The model under review builds one solid part; all positions refer to its coordinate system, in mm. A direction names the side the tool comes from. Round coordinates to 2 decimals unless told otherwise and drop trailing zeros. Order: outer loops, then holes, each group sorted by start corner. A loop starts at its lowest first (then second) coordinate and runs counter-clockwise, first axis right, second up. Notation, with made-up numbers: M 66.25,-0.75 L 110.25,-0.75 A34 ccw 110.25,36.25 Z; hole C 50.25,53.5 d3. An arc over 180 degrees is marked long. Answer as a JSON object with one key per item and string values. Group by question number.
1) Consider section A-A, the plane z = 0. Write out the cut boundary in (x, y), then the cut area to 3 significant figures.
2) Consider section B-B, the plane y = 2. Count the separate pieces of the cut face and the enclosed holes in it, then the cut area to 3 significant figures.
3) Insertion check: pin 1 Ø2 at (x, z) = (1.5, 25.5) entering from -Y; pin 2 Ø0.9 at (y, z) = (2, 28) entering from -X; pin 3 Ø5 at (y, z) = (4.5, 22.5) entering from +X; pin 4 Ø5 at (x, z) = (0.5, 18) entering from +Y. Each pin has a flat end and moves straight along its axis. Give the tip position at first contact, or say it passes through.
4) Consider section D-D, the plane x = -3.5. Write out the cut boundary in (y, z).
5) Consider section C-C, the plane z = 28. Write out the cut boundary in (x, y).
6) To check wall thickness, follow line 1 (X direction, y = 1.05, z = 0); line 2 (Z direction, x = 1.4, y = 2); line 3 (Z direction, x = 0.6, y = 2). State the ranges of each line that lie inside material, in increasing order.
7) For faces 1 (the flat face through (-1.75, 4, 11)), 2 (the flat face through (0, 7, 2)), 3 (the cylindrical face through (1.01, 4.05, 26.53)), list the 3-axis set-ups (+Z, -Z, +X, -X, +Y, -Y) from which the entire face can be reached by the end or side of a thin tool; tool diameter is ignored.
8) The part is to be moulded in two halves that separate along X. For faces 4 (the flat face through (1.75, 3, 17)), 5 (the cylindrical face through (0.173, 1.479, -4.497)), 6 (the cylindrical face through (-0.97, 8.48, -1.27)), 7 (the cylindrical face through (-0.97, 1.48, -1.27)), say which applies: +X half, -X half, draft (parallel to the pull), parting line (faces both ways), or undercut.
```python
from build123d import *

# Parameters (mm, degrees)
SKETCH4_R           = 4.5
SKETCH4_R_2         = 1.6
BOSS_EXTRUDE3_DEPTH = 3
BOSS_EXTRUDE4_START = 4
SKETCH5_R           = 4.5
SKETCH5_R_2         = 1.6
BOSS_EXTRUDE4_DEPTH = 3
BOSS_EXTRUDE5_START = -10
BOSS_EXTRUDE5_DEPTH = 10
CUT_EXTRUDE1_DEPTH  = 17.126453423
SKETCH8_W           = 3.5
SKETCH8_H           = 4
BOSS_EXTRUDE6_DEPTH = 17
SKETCH9_R           = 0.75
CUT_EXTRUDE2_DEPTH  = 31.381943651
SKETCH10_R          = 2.25
SKETCH10_R_2        = 0.75
BOSS_EXTRUDE7_DEPTH = 1.5
FILLET1_R           = 10
FILLET2_R           = 10
FILLET3_R           = 1
SKETCH11_W          = 2
SKETCH11_H          = 2.46221445
CUT_EXTRUDE3_DEPTH  = 33.176272314
CHAMFER2_SIZE       = 4
CHAMFER2_SIZE2      = 1.616104903
CHAMFER3_SIZE       = 0.38
CHAMFER3_SIZE_2     = 1.044041419


with BuildPart() as part:
    # Sketch4 → Boss-Extrude3 (new body)
    with BuildSketch(Plane(origin=(0, 0, 0), x_dir=(1, 0, 0), z_dir=(0, 1, 0))):
        with Locations(Location((0, 0, 0), (0, 0, 270))):
            Circle(SKETCH4_R)
        with Locations(Location((0, 0, 0), (0, 0, 270))):
            Circle(SKETCH4_R_2, mode=Mode.SUBTRACT)
    extrude(amount=BOSS_EXTRUDE3_DEPTH)



with BuildPart() as body_2:
    # Sketch5 → Boss-Extrude4 (new body)
    with BuildSketch(Plane(origin=(0, 3, 0), x_dir=(1, 0, 0), z_dir=(0, 1, 0)).offset(BOSS_EXTRUDE4_START)):
        with Locations(Location((0, 0, 0), (0, 0, 270))):
            Circle(SKETCH5_R)
        with Locations(Location((0, 0, 0), (0, 0, 270))):
            Circle(SKETCH5_R_2, mode=Mode.SUBTRACT)
    extrude(amount=BOSS_EXTRUDE4_DEPTH)


with BuildPart() as part_1:
    add(part.part)

    add(body_2.part)  # Boss-Extrude5 merges body 2
    # Sketch6 → Boss-Extrude5 (add)
    with BuildSketch(Plane(origin=(0, 10, 0), x_dir=(1, 0, 0), z_dir=(0, 1, 0)).offset(BOSS_EXTRUDE5_START)):
        with BuildLine():
            ThreePointArc((1.75, -4.145780988), (0, -4.5), (-1.75, -4.145780988))
            Line((-1.75, -4.145780988), (-1.75, -11))
            Line((-1.75, -11), (1.75, -11))
            Line((1.75, -11), (1.75, -4.145780988))
        make_face()
    extrude(amount=BOSS_EXTRUDE5_DEPTH)

    # Sketch7 → Cut-Extrude1 (cut, through all)
    with BuildSketch(Plane.ZY.offset(1.75)):
        Polygon((4.145780988, 7), (4.145780988, 3), (7.145780988, 3), (9.145780988, 5), (7.145780988, 7), align=None)
    extrude(amount=-CUT_EXTRUDE1_DEPTH, mode=Mode.SUBTRACT)

    # Sketch8 → Boss-Extrude6 (add)
    with BuildSketch(Plane.XY.offset(11)):
        with Locations((0, 2)):
            Rectangle(SKETCH8_W, SKETCH8_H)
    extrude(amount=BOSS_EXTRUDE6_DEPTH)

    # Sketch9 → Cut-Extrude2 (cut, through all)
    with BuildSketch(Plane(origin=(1.75, 0, 0), x_dir=(0, 0, -1), z_dir=(1, 0, 0))):
        with Locations((-28, 2)):
            Circle(SKETCH9_R)
    extrude(amount=-CUT_EXTRUDE2_DEPTH, mode=Mode.SUBTRACT)

    # Sketch10 → Boss-Extrude7 (add)
    with BuildSketch(Plane(origin=(1.75, 0, 0), x_dir=(0, 0, -1), z_dir=(1, 0, 0))):
        with Locations((-28, 2)):
            Circle(SKETCH10_R)
        with Locations((-28, 2)):
            Circle(SKETCH10_R_2, mode=Mode.SUBTRACT)
    extrude(amount=-BOSS_EXTRUDE7_DEPTH)

    # Fillet1
    # the kernel refuses this fillet: 10 mm, written as the material it adds along each edge
    with BuildSketch(Plane(origin=(1.75, 4, 11), x_dir=(0, 1, 0), z_dir=(-1, 0, 0))) as fillet1_piece_1:
        with BuildLine():
            CenterArc((10, -9.16515139), FILLET1_R, 113.578178478, 66.421821522)
            Line((0, -9.16515139), (0, 0))
            Line((0, 0), (6, 0))
        make_face()
    extrude(amount=3.5)
    with BuildSketch(Plane(origin=(0.25, 4, 26.969223594), x_dir=(0, 0, -1), z_dir=(1, 0, 0))) as fillet1_piece_2:
        with BuildLine():
            CenterArc((1.431438044, 10), FILLET1_R, 258.404727341, 11.595272659)
            ThreePointArc((-0.578532936, 0.204081633), (-0.282278366, 0.121850768), (0, 0))
            Line((0, 0), (1.431438044, 0))
        make_face()
    extrude(amount=1.5)
    with BuildSketch(Plane(origin=(0.25, 0, 26.969223594), x_dir=(0, -0.33266579589081224, 0.9430447859165186), z_dir=(1, 0, 0))) as fillet1_piece_3:
        with BuildLine():
            CenterArc((1.976747775, 9.906638335), FILLET1_R, 250.569341445, 11.595272659)
            Line((-1.349910184, 0.476190476), (0, 0))
            ThreePointArc((0, 0), (0.306736724, 0.021006375), (0.613473447, 0))
        make_face()
    extrude(amount=1.5)

    # Fillet2
    fillet2_edges = [part_1.edges().sort_by_distance(p)[0] for p in [
        (0, 10, 11),
    ]]
    fillet(fillet2_edges, radius=FILLET2_R)

    # Fillet3
    fillet3_edges = [part_1.edges().sort_by_distance(p)[0] for p in [
        (0, 7, 7.145780988),
        (0, 5, 9.145780988),
        (0, 3, 7.145780988),
    ]]
    fillet(fillet3_edges, radius=FILLET3_R)

    # Sketch11 → Cut-Extrude3 (cut, through all)
    with BuildSketch(Plane.XZ):
        with Locations((-0.75, 26.768892775)):
            Rectangle(SKETCH11_W, SKETCH11_H)
    extrude(amount=-CUT_EXTRUDE3_DEPTH, mode=Mode.SUBTRACT)

    # Chamfer2
    chamfer2_edges = [part_1.edges().sort_by_distance(p)[0] for p in [
        (-1.75, 2, 25.53778555),
    ]]
    chamfer2_side = [part_1.faces().sort_by_distance(p)[0] for p in [
        (-1.75, 3.550024841, 13.432455859),
    ]]
    chamfer(chamfer2_edges, length=CHAMFER2_SIZE, length2=CHAMFER2_SIZE2, reference=chamfer2_side[0])

    # Chamfer3
    # the kernel refuses this chamfer: 1.044041419, 0.38 mm, written as the material it adds along each edge
    with BuildSketch(Plane(origin=(0.25, -2.708446751, 25.53778555), x_dir=(-0.9950833631817484, 0, -0.09904090225205131), z_dir=(0, 1, 0))) as chamfer3_piece_1_section:
        Polygon((CHAMFER3_SIZE * 0.995083363182, CHAMFER3_SIZE * 0.0990409022521), (-CHAMFER3_SIZE_2 * 0.0990409022893, CHAMFER3_SIZE_2 * 0.995083363556), (0, 0), align=None)
    chamfer3_piece_1 = extrude(amount=9.416893502, mode=Mode.PRIVATE)
    chamfer3_piece_1 = chamfer3_piece_1 - Plane(origin=(0.195523629, 14, 25.53778555), x_dir=(0, 0, -1), z_dir=(-1, 0, 0)) * Cylinder(10, 23, mode=Mode.PRIVATE)
    chamfer3_piece_1 = chamfer3_piece_1 - Plane(origin=(0.195523629, -10, 25.53778555), x_dir=(0, -0.3326657958908282, 0.943044785916513), z_dir=(-1, 0, 0)) * Cylinder(10, 23, mode=Mode.PRIVATE)
    add(chamfer3_piece_1)


solid = part_1.part
```
Results list:
{
 "1": {"outline": "M -4.5,0 L -1.6,0 L -1.6,3 L -4.5,3 Z; M -4.5,7 L -1.6,7 L -1.6,10 L -4.5,10 Z; M 1.6,0 L 4.5,0 L 4.5,3 L 1.6,3 Z; M 1.6,7 L 4.5,7 L 4.5,10 L 1.6,10 Z", "area": "34.8 mm^2"},
 "2": {"separate pieces": "2", "enclosed holes": "1", "area": "131 mm^2"},
 "3": {"pin 1": "y = -0.05", "pin 2": "through", "pin 3": "x = 1.75", "pin 4": "y = 5.15"},
 "4": {"outline": "M 0,-2.83 L 3,-2.83 L 3,2.83 L 0,2.83 Z; M 7,-2.83 L 10,-2.83 L 10,2.83 L 7,2.83 Z"},
 "5": {"outline": "M 0.25,-0.25 L 1.75,-0.25 L 1.75,1.25 L 0.25,1.25 Z; M 0.25,2.75 L 1.75,2.75 L 1.75,4.25 L 0.25,4.25 Z"},
 "6": {"line 1": "-4.5 to -1.6, 1.6 to 4.5", "line 2": "-4.28 to -0.77, 0.77 to 27.25, 28.75 to 30.25", "line 3": "-4.46 to -1.48, 1.48 to 27.25, 28.75 to 30.25"},
 "7": {"face 1": "+Z, -X, +Y, -Y", "face 2": "-Z, +X, -X", "face 3": "+X, -X, +Y"},
 "8": {"face 4": "+X half", "face 5": "parting line", "face 6": "undercut", "face 7": "undercut"}
}
